Verification items for the finished model (mm, model axes). Round coordinates to 2 decimals unless told otherwise and drop trailing zeros. Write each loop counter-clockwise with the first axis right and the second up, starting at its lowest first coordinate (ties: lowest second). Pieces come first, ordered by that corner, then holes. Notation, with made-up numbers: (61, 53.25) -> (107, 53.25) arc R28 ccw to (107, 83.25) -> close; hole circle Ø3 at (-18.5, 35.5). An arc over 180 degrees is marked (long way). Answer as a JSON object with one key per item and string values. Group by question number.
(1) Sectioned sample at C-C on y = 5.1. Count the separate pieces of the cut face and the enclosed holes in it, and give its area (3 significant figures).
(2) Sectioned sample at A-A on x = 0. Record the cut outline in (y, z), and give its area (3 significant figures).
(3) Sectioned sample at D-D on x = 140. Record the cut outline in (y, z).
(4) Gauge pin test, flat ends, axial feed: pin 1 Ø3 at (x, y) = (116, 2) entering from -Z; pin 2 Ø1.5 at (x, y) = (-112, 1.5) entering from +Z; pin 3 Ø1.5 at (x, y) = (119.5, 4.5) entering from -Z. Record the tip position at first contact, or that the pin passes through.
(5) Scan lines: L1, parallel to X at y = 4.35, z = 0; L2, parallel to Z at x = 30, y = 1.95; L3, parallel to X at y = 1.5, z = -64. Record each from-to range of solid material in increasing order. Write a range as from..to.
(6) Sectioned sample at B-B on z = 0. Record the cut outline in (x, y), and give its area (3 significant figures).
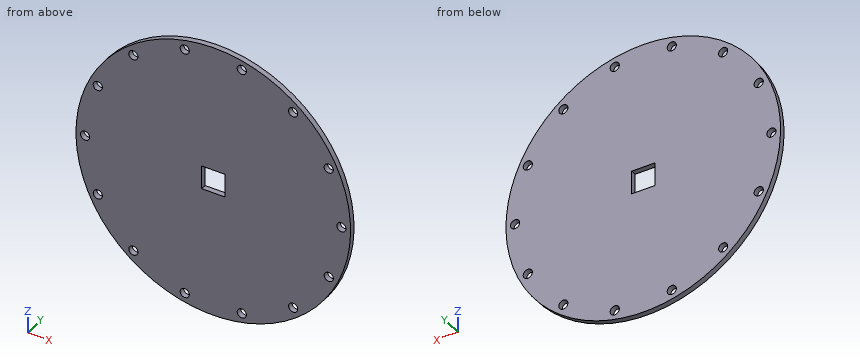
```python
from build123d import *

# Parameters (mm, degrees)
CROQUIS1_R              = 150
SALIENTE_EXTRUIR1_DEPTH = 6
CROQUIS2_R              = 5
CORTAR_EXTRUIR1_DEPTH   = 213.216870206
CROQUIS4_W              = 25.4
CROQUIS4_H              = 25.4
CORTAR_EXTRUIR2_DEPTH   = 213.216870206


with BuildPart() as part:
    # Croquis1 → Saliente-Extruir1 (new body)
    with BuildSketch(Plane(origin=(0, 0, 0), x_dir=(1, 0, 0), z_dir=(0, 1, 0))):
        with Locations(Location((0, 0, 0), (0, 0, 270))):
            Circle(CROQUIS1_R)
    extrude(amount=SALIENTE_EXTRUIR1_DEPTH)

    # Croquis2 → Cortar-Extruir1 (cut, through all)
    with BuildSketch(Plane.XZ):
        with Locations(Location((140, 0, 0), (0, 0, 270))):
            Circle(CROQUIS2_R)
        with Locations(Location((126.135641506, -60.743723476, 0), (0, 0, 270))):
            Circle(CROQUIS2_R)
        with Locations(Location((87.28857226, -109.456407546, 0), (0, 0, 270))):
            Circle(CROQUIS2_R)
        with Locations(Location((31.152930754, -136.489907705, 0), (0, 0, 270))):
            Circle(CROQUIS2_R)
        with Locations(Location((-31.152930754, -136.489907705, 0), (0, 0, 270))):
            Circle(CROQUIS2_R)
        with Locations(Location((-87.28857226, -109.456407546, 0), (0, 0, 270))):
            Circle(CROQUIS2_R)
        with Locations(Location((-126.135641506, -60.743723476, 0), (0, 0, 270))):
            Circle(CROQUIS2_R)
        with Locations(Location((-140, 0, 0), (0, 0, 270))):
            Circle(CROQUIS2_R)
        with Locations(Location((-126.135641506, 60.743723476, 0), (0, 0, 270))):
            Circle(CROQUIS2_R)
        with Locations(Location((-87.28857226, 109.456407546, 0), (0, 0, 270))):
            Circle(CROQUIS2_R)
        with Locations(Location((-31.152930754, 136.489907705, 0), (0, 0, 270))):
            Circle(CROQUIS2_R)
        with Locations(Location((31.152930754, 136.489907705, 0), (0, 0, 270))):
            Circle(CROQUIS2_R)
        with Locations(Location((87.28857226, 109.456407546, 0), (0, 0, 270))):
            Circle(CROQUIS2_R)
        with Locations(Location((126.135641506, 60.743723476, 0), (0, 0, 270))):
            Circle(CROQUIS2_R)
    extrude(amount=-CORTAR_EXTRUIR1_DEPTH, mode=Mode.SUBTRACT)

    # Croquis4 → Cortar-Extruir2 (cut, through all)
    with BuildSketch(Plane.XZ):
        Rectangle(CROQUIS4_W, CROQUIS4_H)
    extrude(amount=-CORTAR_EXTRUIR2_DEPTH, mode=Mode.SUBTRACT)


solid = part.part
```
Computed values:
{
 "1": {"separate pieces": "1", "enclosed holes": "15", "area": "68,900 mm2"},
 "2": {"outline": "(0, -150) -> (6, -150) -> (6, -12.7) -> (0, -12.7) -> close; (0, 12.7) -> (6, 12.7) -> (6, 150) -> (0, 150) -> close", "area": "1,650 mm2"},
 "3": {"outline": "(0, -53.85) -> (6, -53.85) -> (6, -5) -> (0, -5) -> close; (0, 5) -> (6, 5) -> (6, 53.85) -> (0, 53.85) -> close"},
 "4": {"pin 1": "z = -96.9", "pin 2": "z = 100.62", "pin 3": "z = -91.64"},
 "5": {"L1": "-150..-145, -135..-12.7, 12.7..135, 145..150", "L2": "-146.97..-141.36, -131.62..131.62, 141.36..146.97", "L3": "-135.66..-129.93, -122.34..122.34, 129.93..135.66"},
 "6": {"outline": "(-150, 0) -> (-145, 0) -> (-145, 6) -> (-150, 6) -> close; (-135, 0) -> (-12.7, 0) -> (-12.7, 6) -> (-135, 6) -> close; (12.7, 0) -> (135, 0) -> (135, 6) -> (12.7, 6) -> close; (145, 0) -> (150, 0) -> (150, 6) -> (145, 6) -> close", "area": "1,530 mm2"}
}
